from build123d import *

# Parameters (mm, degrees)
SKETCH_1_R      = 1
EXTRUDE_1_DEPTH = 1.5


with BuildPart() as part:
    # 草图1 → 凸台-拉伸1 (new body)
    with BuildSketch(Plane.XY):
        with BuildLine():
            Line((28.670799108, 2), (40, 2))
            ThreePointArc((40, 2), (42, 0), (40, -2))
            Line((40, -2), (28.670799108, -2))
            ThreePointArc((28.670799108, -2), (27.256585545, -1.414213562), (26.670799108, 0))
            Line((26.670799108, 0), (26.670799108, 3))
            ThreePointArc((26.670799108, 3), (24.670799108, 5), (22.670799108, 3))
            Line((22.670799108, 3), (22.670799108, 0))
            ThreePointArc((22.670799108, 0), (22.08501267, -1.414213562), (20.670799108, -2))
            Line((20.670799108, -2), (0, -2))
            ThreePointArc((0, -2), (-2, 0), (0, 2))
            Line((0, 2), (20.670799108, 2))
            Line((20.670799108, 2), (20.670799108, 3))
            ThreePointArc((20.670799108, 3), (24.670799108, 7), (28.670799108, 3))
            Line((28.670799108, 3), (28.670799108, 2))
        make_face()
        with Locations((40, 0)):
            Circle(SKETCH_1_R, mode=Mode.SUBTRACT)
        Circle(SKETCH_1_R, mode=Mode.SUBTRACT)
    extrude(amount=EXTRUDE_1_DEPTH)


solid = part.part
Read the model definition and answer for the solid it produces. Units are mm, in the model's axes. A direction names the side the tool comes from. Give positions to 0.01 mm unless a question says otherwise; leave off trailing zeros. Write each loop counter-clockwise with the first axis right and the second up, starting at its lowest first coordinate (ties: lowest second). Pieces come first, ordered by that corner, then holes. Notation, with made-up numbers: (18, 58.25) - (70, 58.25) arc R24 cw to (70, 90.25) - close; hole circle Ø3 at (13.5, -8). An arc over 180 degrees is marked (long way). Answer in a Markdown table with one row per item. Add a question column.
Item 1: Find the intervals of material crossed by L1, parallel to Y at x = 40, z = 0.45; L2, parallel to X at y = 3, z = 0.6; L3, parallel to Y at x = 13, z = 0.4, in increasing order.
Item 2: Section B-B, the plane x = 31 is taken. Write down the section's boundary in (y, z), and give its area (3 significant figures).
Item 3: Determine the mould class of faces 1 (the face through (10, 2, 1)), 2 (the face through (20.671, 2.5, 0.7)), 3 (the face through (26.671, 1, 1)) for opening direction X: pulls with the +X half, pulls with the -X half, needs draft (parallel to the pull), parting line crosses it, or undercut.
Item 4: Flat-ended cylindrical pins translate along their axes: P1, Ø0.5, axis at y = 2.5, z = 1, coming from the +X side; P2, Ø0.8, axis at x = 5, z = 0.5, coming from the +Y side. Find the tip coordinate at first contact, or state that the pin passes through.
Item 5: Section A-A, the plane z = 1.1 is taken. Write down the section's boundary in (x, y).
Item 6: A tool of negligible diameter and unlimited length cuts with its end or side. For faces 4 (the face through (27.27, -1.43, 0.74)), 5 (the face through (24.6, 7, 0.7)), 6 (the face through (34, 2, 1)), from which of +Z, -Z, +X, -X, +Y, -Y can it reach the whole face along a straight path? Write none if from no direction.
Recorded:
| question | item | result |
|---|---|---|
| 1 | L1 | y = -2 to -1, 1 to 2 |
| 1 | L2 | x = 20.67 to 22.67, 26.67 to 28.67 |
| 1 | L3 | y = -2 to 2 |
| 2 | outline | (-2, 0) - (2, 0) - (2, 1.5) - (-2, 1.5) - close |
| 2 | area | 6.00 mm2 |
| 3 | face 1 | needs draft |
| 3 | face 2 | pulls with the -X half |
| 3 | face 3 | undercut |
| 4 | P1 | stops at x = 28.67 |
| 4 | P2 | stops at y = 2 |
| 5 | outline | (0, -2) - (20.67, -2) arc R2 ccw to (22.67, 0) - (22.67, 3) arc R2 cw to (26.67, 3) - (26.67, 0) arc R2 ccw to (28.67, -2) - (40, -2) arc R2 ccw to (40, 2) - (28.67, 2) - (28.67, 3) arc R4 ccw to (20.67, 3) - (20.67, 2) - (0, 2) arc R2 ccw to start; hole circle Ø2 at (0, 0); hole circle Ø2 at (40, 0) |
| 6 | face 4 | +Z, -Z, -Y |
| 6 | face 5 | +Z, -Z, +Y |
| 6 | face 6 | +Z, -Z, +X, +Y |
